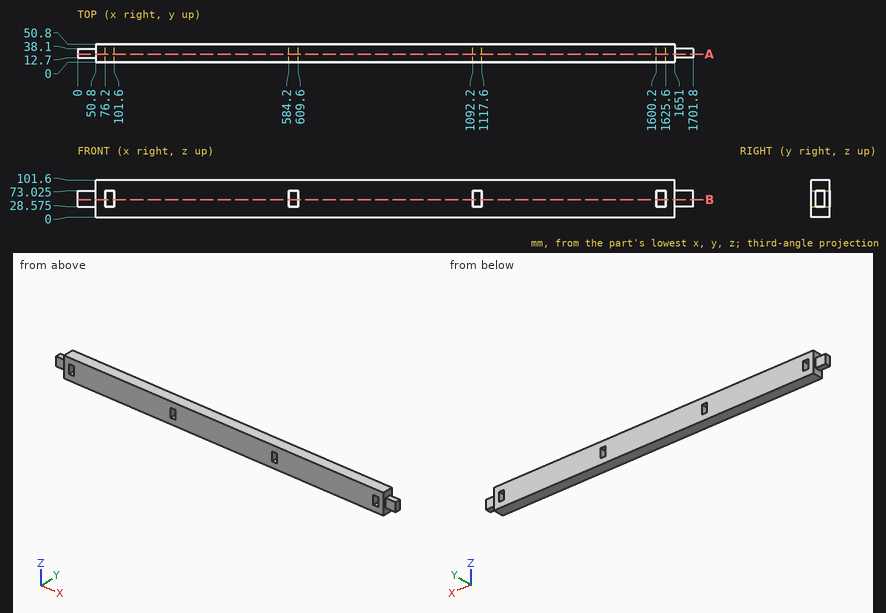
Could you check a few things on this drawing? It's one solid part, dimensions in mm from its lowest x, y, z. Give positions to 0.01 mm unless a question says otherwise; leave off trailing zeros. Write each loop counter-clockwise with the first axis right and the second up, starting at its lowest first coordinate (ties: lowest second). Pieces come first, ordered by that corner, then holes. Notation, with made-up numbers: M 1.5,-35 L 29.5,-35 A22 ccw 29.5,-1 Z; hole C 28,-15.75 d6. An arc over 180 degrees is marked long. Put each result on its own line as item: value. Start each with the question number.
Item 1: If we section it at B-B, the plane z = 48.5: Write out the boundary of the cut face in (x, y), then the cut area to 3 significant figures.
Item 2: Will these pins go through, and if not, where does the flat tip stop? pin 1 (1 mm diameter, centred on x = 1196, z = 54, fed in from -Y); pin 2 (22 mm diameter, centred on x = 1682, z = 47, fed in from -Y); pin 3 (7.5 mm diameter, centred on x = 1688, y = 24, fed in from +Z) (3 decimals); pin 4 (1 mm diameter, centred on y = 6.5, z = 33, fed in from +X).
Item 3: I need wall thicknesses on L1, parallel to X at y = 48, z = 37; L2, parallel to X at y = 29.5, z = 55; L3, parallel to X at y = 43, z = 18.5. Which ranges of each line are inside material? Lowest first, please. Write a range as from..to.
Item 4: If we section it at A-A, the plane y = 22.5: Write out the boundary of the cut face in (x, z) (3 decimals).
Values:
1. outline: M 0,12.7 L 50.8,12.7 L 50.8,0 L 76.2,0 L 76.2,50.8 L 50.8,50.8 L 50.8,38.1 L 0,38.1 Z; M 101.6,0 L 584.2,0 L 584.2,50.8 L 101.6,50.8 Z; M 609.6,0 L 1092.2,0 L 1092.2,50.8 L 609.6,50.8 Z; M 1117.6,0 L 1600.2,0 L 1600.2,50.8 L 1117.6,50.8 Z; M 1625.6,0 L 1651,0 L 1651,12.7 L 1701.8,12.7 L 1701.8,38.1 L 1651,38.1 L 1651,50.8 L 1625.6,50.8 Z
1. area: 78,700 mm²
2. pin 1: y = 0
2. pin 2: y = 12.7
2. pin 3: z = 73.025
2. pin 4: x = 1651
3. L1: 50.8..76.2, 101.6..584.2, 609.6..1092.2, 1117.6..1600.2, 1625.6..1651
3. L2: 0..76.2, 101.6..584.2, 609.6..1092.2, 1117.6..1600.2, 1625.6..1701.8
3. L3: 50.8..1651
4. outline: M 0,28.575 L 50.8,28.575 L 50.8,0 L 1651,0 L 1651,28.575 L 1701.8,28.575 L 1701.8,73.025 L 1651,73.025 L 1651,101.6 L 50.8,101.6 L 50.8,73.025 L 0,73.025 Z; hole M 76.2,28.575 L 101.6,28.575 L 101.6,73.025 L 76.2,73.025 Z; hole M 584.2,28.575 L 609.6,28.575 L 609.6,73.025 L 584.2,73.025 Z; hole M 1092.2,28.575 L 1117.6,28.575 L 1117.6,73.025 L 1092.2,73.025 Z; hole M 1600.2,28.575 L 1625.6,28.575 L 1625.6,73.025 L 1600.2,73.025 Z
